from build123d import *

# Parameters (mm, degrees)
SKETCH1_R           = 2.25
SKETCH1_R_2         = 2.37266458
SKETCH1_W           = 19.08
SKETCH1_H           = 6.38
BOSS_EXTRUDE1_DEPTH = 6.25
SKETCH13_W          = 12.867541265
SKETCH13_H          = 5.004043825
CUT_EXTRUDE1_DEPTH  = 10
CHAMFER1_SIZE       = 10


with BuildPart() as part:
    # Sketch1 → Boss-Extrude1 (new, symmetric)
    with BuildSketch(Plane.XY):
        with BuildLine():
            Line((0, 5), (40, 5))
            Line((40, 5), (40, -5))
            Line((40, -5), (0, -5))
            ThreePointArc((0, -5), (-5, 0), (0, 5))
        make_face()
        Circle(SKETCH1_R, mode=Mode.SUBTRACT)
        with Locations((17.802904034, -0.066795827)):
            Circle(SKETCH1_R_2, mode=Mode.SUBTRACT)
        with Locations((30.033910385, 0.039223356)):
            Rectangle(SKETCH1_W, SKETCH1_H, mode=Mode.SUBTRACT)
    extrude(amount=BOSS_EXTRUDE1_DEPTH, both=True)

    # Sketch13 → Cut-Extrude1 (cut)
    with BuildSketch(Plane.XZ.offset(5)):
        with Locations((1.190063179, -0.07942928)):
            Rectangle(SKETCH13_W, SKETCH13_H)
    extrude(amount=-CUT_EXTRUDE1_DEPTH, mode=Mode.SUBTRACT)

    # Chamfer1
    chamfer1_edges = [part.edges().sort_by_distance(p)[0] for p in [
        (7.623833811, -5, -0.07942928),
    ]]
    chamfer(chamfer1_edges, length=CHAMFER1_SIZE - 0.0001)  # a hair under: the kernel refuses the full size


solid = part.part
Geometry check sheet. Reference: the model listing, model coordinates, mm. A direction names the side the tool comes from. Give positions to 0.01 mm unless a question says otherwise; leave off trailing zeros. Loops run counter-clockwise (first coordinate to the right, second up) from the corner with the lowest first, then second, coordinate; pieces in that order, holes last.
(1) Set-up check for faces 1 (the cylindrical face through (-5, 0, -4)), 2 (the flat face through (20.494, 0, 0)), 3 (the flat face through (6, 0, -2.581)): record each of +Z, -Z, +X, -X, +Y, -Y from which the full face is reachable in a straight line by a thin tool's end or side.
From the geometry:
face 1: +Z, -Z, -X
face 2: +Z, -Z
face 3: -X, -Y
(2) Section check B-B on y = -0.75. Record the cut outline in (x, z).
From the geometry:
outline: (-4.94, -6.25) - (-2.12, -6.25) - (-2.12, -2.58) - (-4.94, -2.58) - close; (-4.94, 2.42) - (-2.12, 2.42) - (-2.12, 6.25) - (-4.94, 6.25) - close; (2.12, -6.25) - (15.53, -6.25) - (15.53, 6.25) - (2.12, 6.25) - (2.12, 2.42) - (13.37, 2.42) - (13.37, -2.58) - (2.12, -2.58) - close; (20.08, -6.25) - (20.49, -6.25) - (20.49, 6.25) - (20.08, 6.25) - close; (39.57, -6.25) - (40, -6.25) - (40, 6.25) - (39.57, 6.25) - close
(3) Depth check by flat-ended pin: pin 1 Ø6 at (x, y) = (0, 0) entering from -Z. Enter the tip coordinate at first touch or a pass-through.
From the geometry:
pin 1: stops at z = -6.25
(4) Section check D-D on y = 4. Record the cut outline in (x, z), then the cut area to 3 significant figures.
From the geometry:
outline: (-3, -6.25) - (40, -6.25) - (40, 6.25) - (-3, 6.25) - (-3, 2.42) - (8.62, 2.42) - (8.62, -2.58) - (-3, -2.58) - close
area: 479 mm2
(5) Section check C-C on z = -3. Record the cut outline in (x, y), then the cut area to 3 significant figures.
From the geometry:
outline: (0, -5) - (40, -5) - (40, 5) - (0, 5) arc R5 ccw to start; hole circle Ø4.5 at (0, 0); hole circle Ø4.75 at (17.8, -0.07); hole (20.49, -3.15) - (39.57, -3.15) - (39.57, 3.23) - (20.49, 3.23) - close
area: 284 mm2
(6) Release check for a two-part mould opening along X. For faces 4 (the flat face through (12.694, -0.07, -0.114)), 5 (the flat face through (6, 0, 2.423)), 6 (the cylindrical face through (-0.29, 2.23, 4.31)), 7 (the flat face through (39.574, 0, 0)) record: released by +X, released by -X, zero draft, split by the parting line, or undercut.
From the geometry:
face 4: released by -X
face 5: zero draft
face 6: undercut
face 7: undercut
(7) Section check A-A on x = 23. Record the cut outline in (y, z), then the cut area to 4 significant figures.
From the geometry:
outline: (-5, -6.25) - (-3.15, -6.25) - (-3.15, 6.25) - (-5, 6.25) - close; (3.23, -6.25) - (5, -6.25) - (5, 6.25) - (3.23, 6.25) - close
area: 45.25 mm2
(8) Thickness scan on L1, parallel to X at y = 0, z = -5.1; L2, parallel to Y at x = 27, z = 2.5; L3, parallel to Y at x = 0, z = 4.2. Record the ranges inside material, lowest first.
From the geometry:
L1: x = -5 to -2.25, 2.25 to 15.43, 20.17 to 20.49, 39.57 to 40
L2: y = -5 to -3.15, 3.23 to 5
L3: y = -5 to -2.25, 2.25 to 5
